The listing builds one solid part. Answer for the finished solid, in the listing's coordinates (mm). Face numbers are marked on the shaded views. Round coordinates to 2 decimals unless told otherwise and drop trailing zeros. Write each loop counter-clockwise with the first axis right and the second up, starting at its lowest first coordinate (ties: lowest second). Pieces come first, ordered by that corner, then holes.
(1) A cutting plane is placed at B-B, the plane x = 68.5. Give the vertices of the cut face in (y, z), and give its area (3 significant figures).
(2) Each of these flat-tipped pins is pushed along its axis until it touches: pin 1 Ø12 at (y, z) = (-58, 67.5) entering from -X; pin 2 Ø10 at (y, z) = (182, 86.5) entering from +X; pin 3 Ø2 at (x, z) = (79, 14.5) entering from +Y. Where does it stop, or does it pass through?
(3) A cutting plane is placed at C-C, the plane y = 147. Give the vertices of the cut face in (x, z).
(4) A cutting plane is placed at D-D, the plane y = 257.5. Give the vertices of the cut face in (x, z).
(5) A cutting plane is placed at A-A, the plane z = 54.5. Give the vertices of the cut face in (x, y).
(6) Find the intervals of material crossed by probe 1 along Y at (x, z) = (0, 71); probe 2 along Y at (x, z) = (-75.5, 6), in increasing order.
(7) The mould has two halves that part along X. Classify the marked faces 1, 2, 3 and 4: +X half, -X half, draft (parallel to the pull), parting line (faces both ways), or undercut.
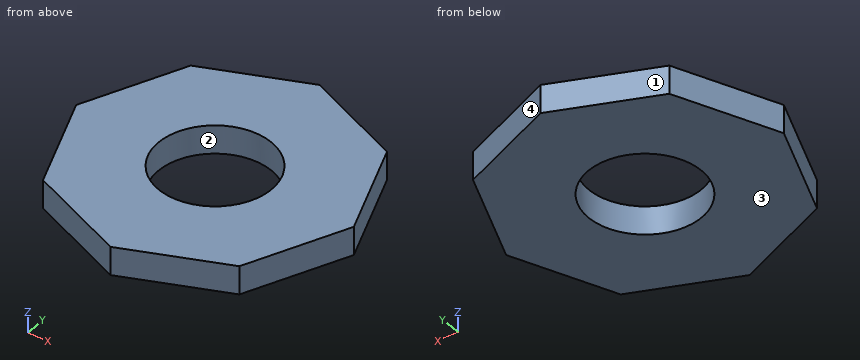
from build123d import *

# Parameters (mm, degrees)
EXTRUDE_1_DEPTH     = 100
SKETCH_2_R          = 200
CUT_EXTRUDE_2_DEPTH = 715.142842854


with BuildPart() as part:
    # 草图1 → 凸台-拉伸1 (new body)
    with BuildSketch(Plane.XY):
        Polygon((500, 0), (353.553390593, 353.553390593), (0, 500), (-353.553390593, 353.553390593), (-500, 0), (-353.553390593, -353.553390593), (0, -500), (353.553390593, -353.553390593), align=None)
    extrude(amount=EXTRUDE_1_DEPTH)

    # 草图2 → 切除-拉伸2 (cut, through all)
    with BuildSketch(Plane.XY):
        Circle(SKETCH_2_R)
    extrude(amount=CUT_EXTRUDE_2_DEPTH, mode=Mode.SUBTRACT)


solid = part.part
Solutions:
1. outline: (-471.63, 0) - (-187.9, 0) - (-187.9, 100) - (-471.63, 100) - close; (187.9, 0) - (471.63, 0) - (471.63, 100) - (187.9, 100) - close
1. area: 56,700 mm2
2. pin 1: stops at x = -478.46
2. pin 2: stops at x = 426.68
2. pin 3: stops at y = 467.69
3. outline: (-439.11, 0) - (-135.61, 0) - (-135.61, 100) - (-439.11, 100) - close; (135.61, 0) - (439.11, 0) - (439.11, 100) - (135.61, 100) - close
4. outline: (-393.34, 0) - (393.34, 0) - (393.34, 100) - (-393.34, 100) - close
5. outline: (-500, 0) - (-353.55, -353.55) - (0, -500) - (353.55, -353.55) - (500, 0) - (353.55, 353.55) - (0, 500) - (-353.55, 353.55) - close; hole circle Ø400 at (0, 0)
6. probe 1: y = -500 to -200, 200 to 500
6. probe 2: y = -468.73 to -185.2, 185.2 to 468.73
7. face 1: -X half
7. face 2: undercut
7. face 3: draft
7. face 4: +X half
